The model under review builds one solid part; all positions refer to its coordinate system, in mm. Face numbers are marked on the shaded views. A direction names the side the tool comes from. Coordinates: 2 decimals unless noted, no trailing zeros. Write each loop counter-clockwise with the first axis right and the second up, starting at its lowest first coordinate (ties: lowest second). Pieces come first, ordered by that corner, then holes. Notation, with made-up numbers: (44.25, 61) - (73.25, 61) arc R20 ccw to (73.25, 100) - close; hole circle Ø8 at (39.25, -1). An arc over 180 degrees is marked (long way). Put each result on its own line as item: value. Start each with the question number.
Item 1: To check wall thickness, follow L1, parallel to Y at x = -8.5, z = 0.75; L2, parallel to X at y = 21, z = 3; L3, parallel to Y at x = -12, z = -1. State the ranges of each line that lie inside material, in increasing order. Write a range as [from, to].
Item 2: Mouldability with a two-part tool opening along X and no side actions: class the marked faces 1, 2 and 3 as pulls with the +X half, pulls with the -X half, needs draft (parallel to the pull), parting line crosses it, or undercut.
Item 3: Consider section B-B on y = 19. Give the boundary of the cut face in (x, z), then the cut area to 3 significant figures.
Item 4: Consider section A-A on x = -4. Give the boundary of the cut face in (y, z), then the cut area to 3 significant figures.
Item 5: Machinability: for the marked faces 4, 5, 6 and 7, which of the approach directions +Z, -Z, +X, -X, +Y, -Y give a long, thin tool a straight path to every point of the face, cutting with its end or side? Answer none if there is none.
Item 6: For pin 1 (3 mm diameter, centred on y = 10, z = 4, fed in from -X); pin 2 (3 mm diameter, centred on x = -8.5, y = 25.5, fed in from +Z); pin 3 (1.2 mm diameter, centred on x = -7, z = 6, fed in from -Y), all flat-tipped, find the tip position at first contact; note any pin that passes through.
Item 7: Consider section C-C on x = -7. Give the boundary of the cut face in (y, z), then the cut area to 3 significant figures.
Item 8: Consider section D-D on z = 3.75. Give the boundary of the cut face in (x, y), then the cut area to 3 significant figures.
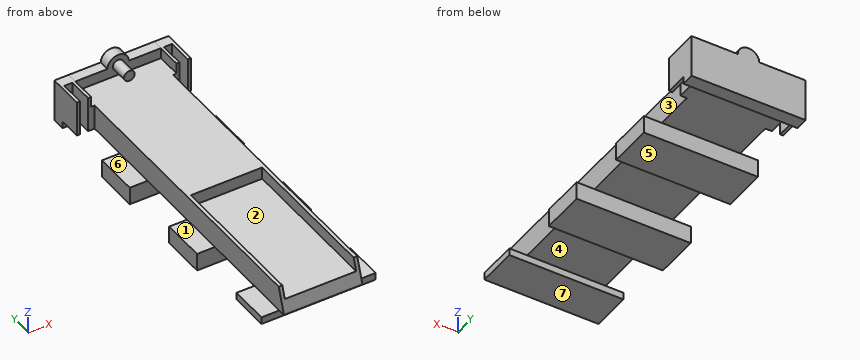
```python
from build123d import *

# Parameters (mm, degrees)
SKETCH2_W            = 14
SKETCH2_H            = 48
BOSS_EXTRUDE1_DEPTH  = 8
SKETCH3_W            = 10
SKETCH3_H            = 3.5
CUT_EXTRUDE1_DEPTH   = 51.635955605
CUT_EXTRUDE4_DEPTH   = 48
CUT_EXTRUDE5_REACH   = 51.933
SKETCH16_W           = 1.002160824
SKETCH16_H           = 48
BOSS_EXTRUDE4_DEPTH  = 1
SKETCH17_W           = 1.002160824
SKETCH17_H           = 48
BOSS_EXTRUDE5_DEPTH  = 1
SKETCH25_W           = 2
SKETCH25_H           = 5
BOSS_EXTRUDE10_DEPTH = 5
SKETCH26_W           = 12
SKETCH26_H           = 1.5
BOSS_EXTRUDE11_DEPTH = 1.5
SKETCH27_R           = 1.5
BOSS_EXTRUDE14_DEPTH = 1.5
SKETCH29_R           = 0.75
CUT_EXTRUDE12_DEPTH  = 1.5
SKETCH30_W           = 1.15
SKETCH30_H           = 3.49
CUT_EXTRUDE13_DEPTH  = 5
SKETCH32_W           = 10
SKETCH32_H           = 47.172433363
BOSS_EXTRUDE15_DEPTH = 3.5
BOSS_EXTRUDE16_DEPTH = 10
SKETCH34_W           = 10
SKETCH34_H           = 20.2
CUT_EXTRUDE15_DEPTH  = 1.7
SKETCH35_W           = 10
SKETCH35_H           = 1.7
CUT_EXTRUDE16_DEPTH  = 1
CUT_EXTRUDE18_START  = -16
SKETCH38_W           = 1.002160824
SKETCH38_H           = 8.4
SKETCH38_H_2         = 8.398563286
CUT_EXTRUDE18_DEPTH  = 16
CUT_EXTRUDE19_DEPTH  = 20
SKETCH43_W           = 16
SKETCH43_H           = 1.002160824
CUT_EXTRUDE20_DEPTH  = 0.4
SKETCH44_W           = 16
SKETCH44_H           = 1.002160824
CUT_EXTRUDE21_DEPTH  = 0.4
SKETCH45_W           = 16
SKETCH45_H           = 1.002160824
CUT_EXTRUDE22_DEPTH  = 0.4
SKETCH46_R           = 0.75
BOSS_EXTRUDE18_DEPTH = 4
SKETCH47_W           = 10
SKETCH47_H           = 1.7
CUT_EXTRUDE23_DEPTH  = 1
CUT_EXTRUDE24_DEPTH  = 0.5
CUT_EXTRUDE25_DEPTH  = 0.5
CUT_EXTRUDE26_DEPTH  = 52.14944604
SKETCH51_W           = 16
SKETCH51_H           = 6.2
BOSS_EXTRUDE19_DEPTH = 2
SKETCH52_W           = 0.5
SKETCH52_H           = 6.2
CUT_EXTRUDE27_DEPTH  = 16
SKETCH53_W           = 0.5
SKETCH53_H           = 6.2
CUT_EXTRUDE28_DEPTH  = 16


with BuildPart() as part:
    # Sketch2 → Boss-Extrude1 (new body)
    with BuildSketch(Plane.XY):
        with Locations((-7, 24)):
            Rectangle(SKETCH2_W, SKETCH2_H)
    extrude(amount=BOSS_EXTRUDE1_DEPTH)

    # Sketch3 → Cut-Extrude1 (cut, through all)
    with BuildSketch(Plane(origin=(0, 0, 0), x_dir=(-1, 0, 0), z_dir=(0, -1, 0))):
        with Locations((7, -1.75)):
            Rectangle(SKETCH3_W, SKETCH3_H)
    extrude(amount=-CUT_EXTRUDE1_DEPTH, mode=Mode.SUBTRACT)

    # Sketch7 → Cut-Extrude4 (cut)
    with BuildSketch(Plane.XZ):
        Polygon((-14, 1.002160824), (-13, 1.002160824), (-13, 4.501055273), (-1, 4.501055273), (-1, 1.002160824), (0, 1.002160824), (0, 8), (-14, 8), align=None)
    extrude(amount=-CUT_EXTRUDE4_DEPTH, mode=Mode.SUBTRACT)

    # Cut-Extrude5: up to this face of the body (flat: up to its plane)
    cut_extrude5_end = Plane(part.part.faces().sort_by_distance((-1, 24, 2.751608048))[0])
    # Sketch9 → Cut-Extrude5 (cut, up to the picked face)
    with BuildSketch(Plane.ZY.offset(13), mode=Mode.PRIVATE) as cut_extrude5_sk1:
        Polygon((1.002160824, 0), (4.501055273, 1.159229281), (4.501055273, 0), align=None)
    cut_extrude5_tool1 = split(extrude(cut_extrude5_sk1.sketch, amount=-CUT_EXTRUDE5_REACH, mode=Mode.PRIVATE), bisect_by=cut_extrude5_end, keep=Keep.BOTH, mode=Mode.PRIVATE)
    add(cut_extrude5_tool1.solids().sort_by(Axis((-13, 0.38641, 3.334757), (1, 0, 0)))[0], mode=Mode.SUBTRACT)

    # Sketch16 → Boss-Extrude4 (add)
    with BuildSketch(Plane(origin=(0, 0, 0), x_dir=(0, 0, -1), z_dir=(1, 0, 0))):
        with Locations((-0.501080412, 24)):
            Rectangle(SKETCH16_W, SKETCH16_H)
    extrude(amount=BOSS_EXTRUDE4_DEPTH)

    # Sketch17 → Boss-Extrude5 (add)
    with BuildSketch(Plane.ZY.offset(14)):
        with Locations((0.501080412, 24)):
            Rectangle(SKETCH17_W, SKETCH17_H)
    extrude(amount=BOSS_EXTRUDE5_DEPTH)

    # Sketch25 → Boss-Extrude10 (add)
    with BuildSketch(Plane.XY.offset(1.002160824)):
        with Locations((0, 45.5)):
            Rectangle(SKETCH25_W, SKETCH25_H)
        with Locations((-14, 45.5)):
            Rectangle(SKETCH25_W, SKETCH25_H)
    extrude(amount=BOSS_EXTRUDE10_DEPTH)

    # Sketch26 → Boss-Extrude11 (add)
    with BuildSketch(Plane.XY.offset(4.501055273)):
        with Locations((-7, 47.25)):
            Rectangle(SKETCH26_W, SKETCH26_H)
    extrude(amount=BOSS_EXTRUDE11_DEPTH)

    # Sketch27 → Boss-Extrude14 (add)
    with BuildSketch(Plane(origin=(0, 48, 0), x_dir=(1, 0, 0), z_dir=(0, 1, 0))):
        with Locations((-7.000000094, -6.001055273)):
            Circle(SKETCH27_R)
    extrude(amount=-BOSS_EXTRUDE14_DEPTH)

    # Sketch29 → Cut-Extrude12 (cut)
    with BuildSketch(Plane(origin=(0, 48, 0), x_dir=(1, 0, 0), z_dir=(0, 1, 0))):
        with Locations(Location((-7.000000094, -6.001055273, 0), (0, 0, 270))):
            Circle(SKETCH29_R)
    extrude(amount=-CUT_EXTRUDE12_DEPTH, mode=Mode.SUBTRACT)

    # Sketch30 → Cut-Extrude13 (cut)
    with BuildSketch(Plane.XY.offset(6.002160824)):
        with Locations((-13.985, 44.745)):
            Rectangle(SKETCH30_W, SKETCH30_H)
        with Locations((-0.015, 44.745)):
            Rectangle(SKETCH30_W, SKETCH30_H)
    extrude(amount=-CUT_EXTRUDE13_DEPTH, mode=Mode.SUBTRACT)

    # Sketch32 → Boss-Extrude15 (add)
    with BuildSketch(Plane(origin=(0, 0, 3.5), x_dir=(-1, 0, 0), z_dir=(0, 0, -1))):
        with Locations((7, 24.413783318)):
            Rectangle(SKETCH32_W, SKETCH32_H)
    extrude(amount=BOSS_EXTRUDE15_DEPTH)

    # Sketch33 → Boss-Extrude16 (add)
    with BuildSketch(Plane(origin=(-12, 0, 0), x_dir=(0, 0, -1), z_dir=(1, 0, 0))):
        Polygon((-3.5, 0.827566637), (0, 0.827566637), (0, -0.332028927), align=None)
    extrude(amount=BOSS_EXTRUDE16_DEPTH)

    # Sketch34 → Cut-Extrude15 (cut)
    with BuildSketch(Plane.XY.offset(4.501055273)):
        with Locations((-7, 11.259229281)):
            Rectangle(SKETCH34_W, SKETCH34_H)
    extrude(amount=-CUT_EXTRUDE15_DEPTH, mode=Mode.SUBTRACT)

    # Sketch35 → Cut-Extrude16 (cut)
    with BuildSketch(Plane(origin=(0, 1.159229281, 0), x_dir=(1, 0, 0), z_dir=(0, 1, 0))):
        with Locations((-7, -3.651055273)):
            Rectangle(SKETCH35_W, SKETCH35_H)
    extrude(amount=-CUT_EXTRUDE16_DEPTH, mode=Mode.SUBTRACT)

    # Sketch38 → Cut-Extrude18 (cut)
    with BuildSketch(Plane(origin=(1, 0, 0), x_dir=(0, 0, -1), z_dir=(1, 0, 0)).offset(CUT_EXTRUDE18_START)):
        with Locations((-0.501080412, 11.591582536)):
            Rectangle(SKETCH38_W, SKETCH38_H)
        with Locations((-0.501080412, 26.591582536)):
            Rectangle(SKETCH38_W, SKETCH38_H)
        with Locations((-0.501080412, 41.590864179)):
            Rectangle(SKETCH38_W, SKETCH38_H_2)
    extrude(amount=CUT_EXTRUDE18_DEPTH, mode=Mode.SUBTRACT)

    # Sketch40 → Cut-Extrude19 (cut)
    with BuildSketch(Plane.ZY.offset(15)):
        Polygon((4.501055273, 1.159229281), (0, -0.332028927), (0, 0.467971073), (4.501055273, 1.959229281), align=None)
    extrude(amount=-CUT_EXTRUDE19_DEPTH, mode=Mode.SUBTRACT)

    # Sketch43 → Cut-Extrude20 (cut)
    with BuildSketch(Plane.XZ.offset(-45.790145822)):
        with Locations((-7, 0.501080412)):
            Rectangle(SKETCH43_W, SKETCH43_H)
    extrude(amount=-CUT_EXTRUDE20_DEPTH, mode=Mode.SUBTRACT)

    # Sketch44 → Cut-Extrude21 (cut)
    with BuildSketch(Plane(origin=(0, 30.791582536, 0), x_dir=(-1, 0, 0), z_dir=(0, -1, 0))):
        with Locations((7, -0.501080412)):
            Rectangle(SKETCH44_W, SKETCH44_H)
    extrude(amount=-CUT_EXTRUDE21_DEPTH, mode=Mode.SUBTRACT)

    # Sketch45 → Cut-Extrude22 (cut)
    with BuildSketch(Plane.XZ.offset(-15.791582536)):
        with Locations((-7, 0.501080412)):
            Rectangle(SKETCH45_W, SKETCH45_H)
    extrude(amount=-CUT_EXTRUDE22_DEPTH, mode=Mode.SUBTRACT)

    # Sketch46 → Boss-Extrude18 (add)
    with BuildSketch(Plane(origin=(0, 48, 0), x_dir=(1, 0, 0), z_dir=(0, 1, 0))):
        with Locations(Location((-7.000000094, -6.001055273, 0), (0, 0, 270))):
            Circle(SKETCH46_R)
    extrude(amount=-BOSS_EXTRUDE18_DEPTH)

    # Sketch47 → Cut-Extrude23 (cut)
    with BuildSketch(Plane.XZ.offset(-21.359229281)):
        with Locations((-7, 3.651055273)):
            Rectangle(SKETCH47_W, SKETCH47_H)
    extrude(amount=-CUT_EXTRUDE23_DEPTH, mode=Mode.SUBTRACT)

    # Sketch48 → Cut-Extrude24 (cut)
    with BuildSketch(Plane(origin=(-1, 0, 0), x_dir=(0, 0, -1), z_dir=(1, 0, 0))):
        Polygon((-4.501055273, 1.959229281), (-1.002160824, 0.8), (-1.002160824, 43), (-4.501055273, 43), align=None)
    extrude(amount=-CUT_EXTRUDE24_DEPTH, mode=Mode.SUBTRACT)

    # Sketch49 → Cut-Extrude25 (cut)
    with BuildSketch(Plane.ZY.offset(13)):
        Polygon((1.002160824, 0.8), (4.501055273, 1.959229281), (4.501055273, 43), (1.002160824, 43), align=None)
    extrude(amount=-CUT_EXTRUDE25_DEPTH, mode=Mode.SUBTRACT)

    # Sketch50 → Cut-Extrude26 (cut, through all)
    with BuildSketch(Plane(origin=(1, 0, 0), x_dir=(0, 0, -1), z_dir=(1, 0, 0))):
        Polygon((-1.002160824, 0.8), (0, 0.467971073), (0, 1.826644399), (-1.002160824, 1.826644399), align=None)
    extrude(amount=-CUT_EXTRUDE26_DEPTH, mode=Mode.SUBTRACT)

    # Sketch51 → Boss-Extrude19 (add)
    with BuildSketch(Plane(origin=(0, 0, 0), x_dir=(-1, 0, 0), z_dir=(0, 0, -1))):
        with Locations((7, 19.291582536)):
            Rectangle(SKETCH51_W, SKETCH51_H)
        with Locations((7, 34.291582536)):
            Rectangle(SKETCH51_W, SKETCH51_H)
    extrude(amount=BOSS_EXTRUDE19_DEPTH)

    # Sketch52 → Cut-Extrude27 (cut)
    with BuildSketch(Plane(origin=(1, 0, 0), x_dir=(0, 0, -1), z_dir=(1, 0, 0))):
        with Locations((1.75, 19.291582536)):
            Rectangle(SKETCH52_W, SKETCH52_H)
    extrude(amount=-CUT_EXTRUDE27_DEPTH, mode=Mode.SUBTRACT)

    # Sketch53 → Cut-Extrude28 (cut)
    with BuildSketch(Plane(origin=(1, 0, 0), x_dir=(0, 0, -1), z_dir=(1, 0, 0))):
        with Locations((1.75, 34.291582536)):
            Rectangle(SKETCH53_W, SKETCH53_H)
    extrude(amount=-CUT_EXTRUDE28_DEPTH, mode=Mode.SUBTRACT)


solid = part.part
```
Report:
1. L1: [1.83, 7.39], [16.19, 22.39], [31.19, 37.39], [46.19, 48]
1. L2: [-12.5, -12], [-2, -1.5]
1. L3: [16.19, 22.39], [31.19, 37.39]
2. face 1: needs draft
2. face 2: undercut
2. face 3: pulls with the +X half
3. outline: (-15, -1.5) - (1, -1.5) - (1, 1) - (-1.5, 1) - (-1.5, 4.5) - (-2, 4.5) - (-2, 2.8) - (-12, 2.8) - (-12, 4.5) - (-12.5, 4.5) - (-12.5, 1) - (-15, 1) - close
3. area: 61.5 mm²
4. outline: (0.8, 1) - (1.83, 1) - (1.83, 0) - (7.39, 0) - (7.39, 1) - (16.19, 1) - (16.19, -1.5) - (22.39, -1.5) - (22.39, 1) - (31.19, 1) - (31.19, -1.5) - (37.39, -1.5) - (37.39, 1) - (46.19, 1) - (46.19, 0) - (48, 0) - (48, 6) - (46.5, 6) - (46.5, 4.5) - (22.36, 4.5) - (22.36, 2.8) - (1.4, 2.8) - close
4. area: 169 mm²
5. face 4: -Z, +X, -X
5. face 5: -Z, +X, -X, +Y, -Y
5. face 6: +Z, -X, -Y
5. face 7: -Z, +X, -X, -Y
6. pin 1: x = -12.5
6. pin 2: z = 4.5
6. pin 3: y = 44
7. outline: (0.8, 1) - (1.83, 1) - (1.83, 0) - (7.39, 0) - (7.39, 1) - (16.19, 1) - (16.19, -1.5) - (22.39, -1.5) - (22.39, 1) - (31.19, 1) - (31.19, -1.5) - (37.39, -1.5) - (37.39, 1) - (46.19, 1) - (46.19, 0) - (48, 0) - (48, 7.5) - (46.5, 7.5) - (46.5, 6.75) - (44, 6.75) - (44, 5.25) - (46.5, 5.25) - (46.5, 4.5) - (22.36, 4.5) - (22.36, 2.8) - (1.4, 2.8) - close
7. area: 175 mm²
8. outline: (-15, 43) - (-14.56, 43) - (-14.56, 46.49) - (-13.41, 46.49) - (-13.41, 43) - (-12.5, 43) - (-12.5, 1.71) - (-12, 1.71) - (-12, 22.36) - (-2, 22.36) - (-2, 1.71) - (-1.5, 1.71) - (-1.5, 43) - (-0.59, 43) - (-0.59, 46.49) - (0.56, 46.49) - (0.56, 43) - (1, 43) - (1, 48) - (-15, 48) - close
8. area: 320 mm²
